Drawing for the job (mm, zero at the part's lowest x, y, z). A direction names the side the tool comes from. Round coordinates to 2 decimals unless told otherwise and drop trailing zeros. Write each loop counter-clockwise with the first axis right and the second up, starting at its lowest first coordinate (ties: lowest second). Pieces come first, ordered by that corner, then holes.
Item 1: Drop flat-ended pins along their axis: pin 1 Ø0.8 at (y, z) = (20, 1.5) entering from -X; pin 2 Ø0.8 at (y, z) = (20.5, 1.5) entering from +X; pin 3 Ø0.8 at (y, z) = (11, 1.5) entering from +X. Give the stop position or say it passes through.
Item 2: Band-saw the part on B-B, the plane y = 4. Write the cut outline in (x, z) (1 decimal).
Item 3: Band-saw the part on A-A, the plane z = 1.3. Write the cut outline in (x, y) (1 decimal), then the cut area to 3 significant figures.
Item 4: Mould opens along Y. For the marked faces 1 and 2 say: +Y half, -Y half, draft (parallel to the pull), parting line (faces both ways), or undercut.
Item 5: Wall check: probe 1 along Y at (x, z) = (13, 1.7) (1 decimal); probe 2 along X at (y, z) = (12.5, 1.9) (1 decimal); probe 3 along Y at (x, z) = (8.75, 1.6) (1 decimal). Give the ranges that are in metal, low to high.
Item 6: 3-axis set-ups, long thin cutter, end or side, ignore diameter. For the marked faces 3, 4 and 5: which of +Z, -Z, +X, -X, +Y, -Y reach the whole face in a straight line?
Item 7: Band-saw the part on D-D, the plane y = 18.5. Write the cut outline in (x, z).
Item 8: Band-saw the part on C-C, the plane x = 13. Write the cut outline in (y, z) (1 decimal).
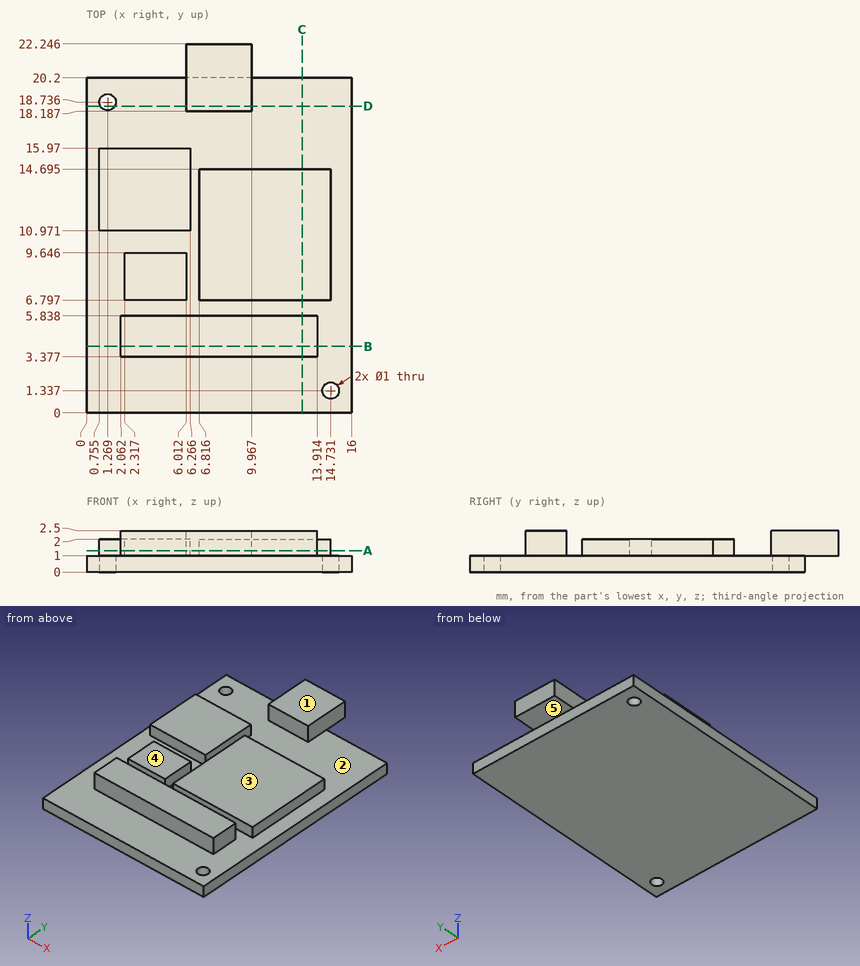
Results:
1. pin 1: stops at x = 6.01
1. pin 2: stops at x = 9.97
1. pin 3: stops at x = 14.73
2. outline: (0, 0) - (16, 0) - (16, 1) - (13.9, 1) - (13.9, 2.5) - (2.1, 2.5) - (2.1, 1) - (0, 1) - close
3. outline: (0.8, 11) - (6.3, 11) - (6.3, 16) - (0.8, 16) - close; (2.1, 3.4) - (13.9, 3.4) - (13.9, 5.8) - (2.1, 5.8) - close; (2.3, 6.8) - (6, 6.8) - (6, 9.6) - (2.3, 9.6) - close; (6, 18.2) - (10, 18.2) - (10, 22.2) - (6, 22.2) - close; (6.8, 6.8) - (14.7, 6.8) - (14.7, 14.7) - (6.8, 14.7) - close
3. area: 146 mm2
4. face 1: draft
4. face 2: undercut
5. probe 1: y = 3.4 to 5.8, 6.8 to 14.7
5. probe 2: x = 0.8 to 6.3, 6.8 to 14.7
5. probe 3: y = 3.4 to 5.8, 6.8 to 14.7, 18.2 to 22.2
6. face 3: +Z, +X, -X
6. face 4: +Z, +X, -X, +Y
6. face 5: -Z, +X, -X, +Y
7. outline: (0, 0) - (0.83, 0) - (0.83, 1) - (0, 1) - close; (1.71, 0) - (16, 0) - (16, 1) - (9.97, 1) - (9.97, 2.5) - (6.01, 2.5) - (6.01, 1) - (1.71, 1) - close
8. outline: (0, 0) - (20.2, 0) - (20.2, 1) - (14.7, 1) - (14.7, 2) - (6.8, 2) - (6.8, 1) - (5.8, 1) - (5.8, 2.5) - (3.4, 2.5) - (3.4, 1) - (0, 1) - close
